Geometry: final body of the model. Coordinates: model frame, mm. Face numbers are marked on the shaded views. Give positions to 0.01 mm unless a question says otherwise; leave off trailing zeros. Loops run counter-clockwise (first coordinate to the right, second up) from the corner with the lowest first, then second, coordinate; pieces in that order, holes last.
from build123d import *

# Parameters (mm, degrees)
F0_W        = 44
F0_H        = 41
F1_DEPTH    = 4
F2_R        = 1.75
F3_DEPTH    = 4.001
F4_R        = 3.25
F5_DEPTH    = 2.5
F6_T1_DEPTH = 46
F6_T3_DEPTH = 49


# Not quite as in the source:
# - a fillet or chamfer that OpenCascade refuses, or shapes differently, is made with other operations: its cross-section is extruded or revolved along the edge and cut away or added


with BuildPart() as f1:
    # F0 (on Top) → F1 (new body)
    with BuildSketch(Plane.XY):
        with Locations((17.9585738778, -18.5538536012)):
            Rectangle(F0_W, F0_H)
    extrude(amount=F1_DEPTH)

    # F2 (on face) → F3 (cut, through all)
    with BuildSketch(Plane.XY.offset(4)):
        with Locations((-0.0414261222, -2.0538536012)):
            Circle(F2_R)
        with Locations((35.9585738778, -2.0538536012)):
            Circle(F2_R)
        with Locations((35.9585738778, -35.0538536012)):
            Circle(F2_R)
        with Locations((-0.0414261222, -35.0538536012)):
            Circle(F2_R)
    extrude(amount=-F3_DEPTH, mode=Mode.SUBTRACT)

    # F4 (on face) → F5 (cut)
    with BuildSketch(Plane.XY.offset(4)):
        with Locations((-0.0414261222, -2.0538536012)):
            Circle(F4_R)
        with Locations((35.9585738778, -2.0538536012)):
            Circle(F4_R)
        with Locations((35.9585738778, -35.0538536012)):
            Circle(F4_R)
        with Locations((-0.0414261222, -35.0538536012)):
            Circle(F4_R)
    extrude(amount=-F5_DEPTH, mode=Mode.SUBTRACT)

    # F6: fillet of radius 1 on 4 edges, made by hand

    # F6_s2 → F6_t1 (cut)
    with BuildSketch(Plane.XZ.offset(-4.4461463988)):
        with BuildLine():
            ThreePointArc((-3.0414261222, 4), (-3.7485329034, 3.7071067812), (-4.0414261222, 3))
            Line((-4.0414261222, 3), (-4.0414261222, 4))
            Line((-4.0414261222, 4), (-3.0414261222, 4))
        make_face()
        with BuildLine():
            ThreePointArc((39.9585738778, 3), (39.665680659, 3.7071067812), (38.9585738778, 4))
            Line((38.9585738778, 4), (39.9585738778, 4))
            Line((39.9585738778, 4), (39.9585738778, 3))
        make_face()
    extrude(amount=F6_T1_DEPTH, mode=Mode.SUBTRACT)

    # F6_s4 → F6_t3 (cut)
    with BuildSketch(Plane.YZ.offset(-6.5414261222)):
        with BuildLine():
            ThreePointArc((-39.0538536012, 3), (-38.7609603824, 3.7071067812), (-38.0538536012, 4))
            Line((-38.0538536012, 4), (-39.0538536012, 4))
            Line((-39.0538536012, 4), (-39.0538536012, 3))
        make_face()
        with BuildLine():
            ThreePointArc((1.9461463988, 3), (1.65325318, 3.7071067812), (0.9461463988, 4))
            Line((0.9461463988, 4), (1.9461463988, 4))
            Line((1.9461463988, 4), (1.9461463988, 3))
        make_face()
    extrude(amount=F6_T3_DEPTH, mode=Mode.SUBTRACT)


solid = f1.part
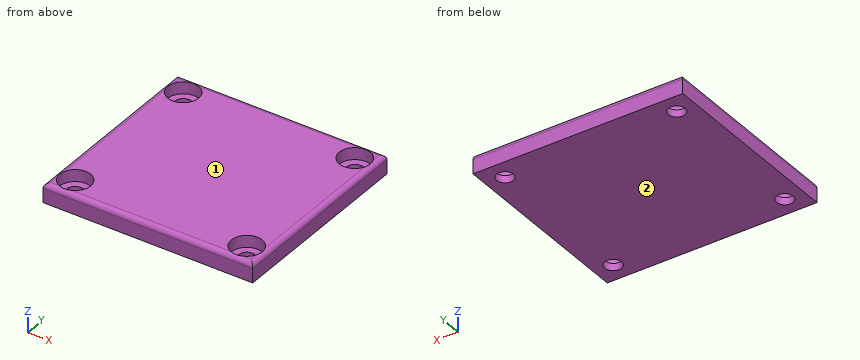
Item 1: Pin query (flat end, axial travel): pin 1 (7 mm diameter, centred on x = -1, y = -1.5, fed in from +Z); pin 2 (2 mm diameter, centred on x = 36, y = -33.5, fed in from +Z). Return the tip coordinate at first contact, or that it passes through.
Values follow:
pin 1: stops at z = 4
pin 2: stops at z = 1.5
Item 2: Draft query along Z for the marked faces 1 and 2. Return one class per face: +Z half, -Z half, draft (parallel to the pull), parting line (faces both ways), or undercut.
Values follow:
face 1: +Z half
face 2: -Z half
Item 3: Section query B-B on x = 0. Return loops of the section in (y, z), plus the area to 3 significant figures.
Values follow:
outline: (-39.05, 0) - (-36.8, 0) - (-36.8, 1.5) - (-38.3, 1.5) - (-38.3, 3.97) arc R1 ccw to (-39.05, 3) - close; (-33.3, 0) - (-3.8, 0) - (-3.8, 1.5) - (-5.3, 1.5) - (-5.3, 4) - (-31.8, 4) - (-31.8, 1.5) - (-33.3, 1.5) - close; (-0.3, 0) - (1.95, 0) - (1.95, 3) arc R1 ccw to (1.2, 3.97) - (1.2, 1.5) - (-0.3, 1.5) - close
area: 121 mm2
Item 4: Section query A-A on z = 2.15. Return loops of the section in (x, y), plus the area to 3 significant figures.
Values follow:
outline: (-4.04, -39.05) - (39.96, -39.05) - (39.96, 1.95) - (-4.04, 1.95) - close; hole circle Ø6.5 at (-0.04, -35.05); hole circle Ø6.5 at (-0.04, -2.05); hole circle Ø6.5 at (35.96, -35.05); hole circle Ø6.5 at (35.96, -2.05)
area: 1,670 mm2
Item 5: Ray query, probe 1 along X at (y, z) = (-1, 2.5); probe 2 along Y at (x, z) = (1.5, 3.45); probe 3 along Y at (x, z) = (-1, 0.75). Return the intervals inside material, ascending.
Values follow:
probe 1: x = -4.04 to -3.12, 3.03 to 32.88, 39.03 to 39.96
probe 2: y = -38.95 to -37.92, -32.19 to -4.92, 0.81 to 1.84
probe 3: y = -39.05 to -36.52, -33.59 to -3.52, -0.59 to 1.95
